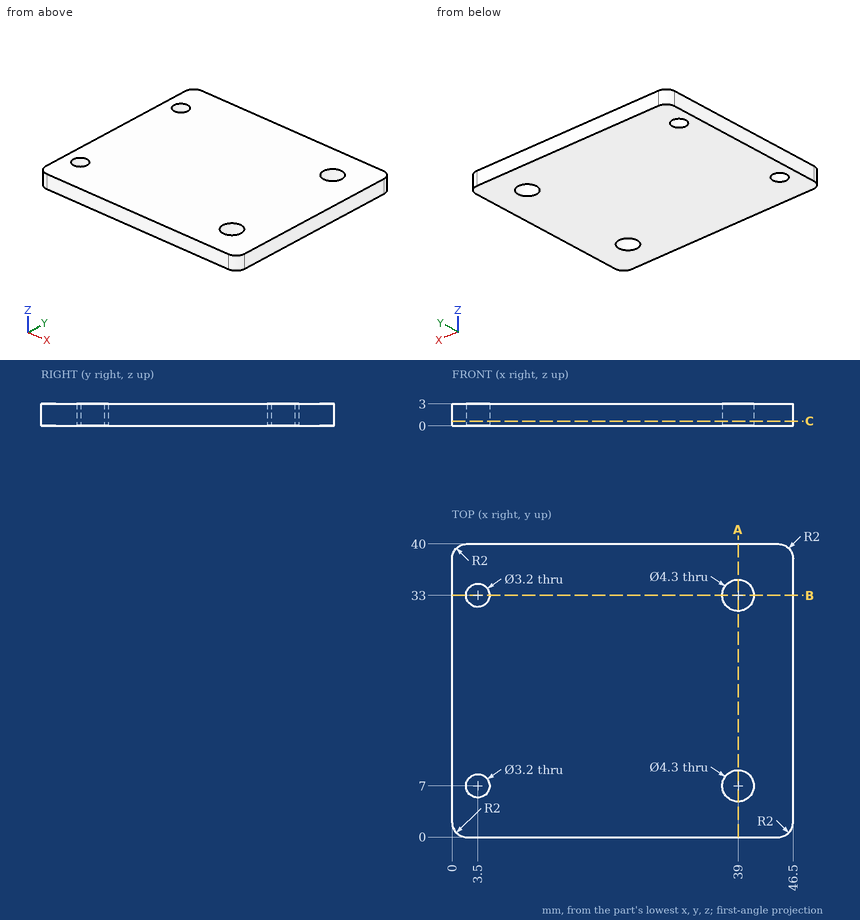
Can you work these out from the drawing? Everything is in mm from the part's minimum corner. Round coordinates to 2 decimals unless told otherwise and drop trailing zeros. Loops run counter-clockwise (first coordinate to the right, second up) from the corner with the lowest first, then second, coordinate; pieces in that order, holes last. Notation, with made-up numbers: (-8, 34.25) -> (0, 34.25) arc R20 ccw to (0, 64.25) -> close; hole circle Ø11 at (-0.75, -9.5). An arc over 180 degrees is marked (long way). One line per question, with ' | ' between items.
(1) If we section it at B-B on y = 33: List the corners of the cut face in (x, z) for me.
Model answer:
outline: (0, 0) -> (1.9, 0) -> (1.9, 3) -> (0, 3) -> close; (5.1, 0) -> (36.85, 0) -> (36.85, 3) -> (5.1, 3) -> close; (41.15, 0) -> (46.5, 0) -> (46.5, 3) -> (41.15, 3) -> close
(2) If I drill on probe 1 along Y at (x, z) = (39, 1.55); probe 2 along Y at (x, z) = (3.5, 0.7); probe 3 along X at (y, z) = (7.5, 0.7), over which ranges is the centre line in solid material (lowest first)?
Model answer:
probe 1: y = 0 to 4.85, 9.15 to 30.85, 35.15 to 40 | probe 2: y = 0 to 5.4, 8.6 to 31.4, 34.6 to 40 | probe 3: x = 0 to 1.98, 5.02 to 36.91, 41.09 to 46.5
(3) If we section it at C-C on z = 0.65: List the corners of the cut face in (x, y) for me.
Model answer:
outline: (0, 2) arc R2 ccw to (2, 0) -> (44.5, 0) arc R2 ccw to (46.5, 2) -> (46.5, 38) arc R2 ccw to (44.5, 40) -> (2, 40) arc R2 ccw to (0, 38) -> close; hole circle Ø3.2 at (3.5, 7); hole circle Ø3.2 at (3.5, 33); hole circle Ø4.3 at (39, 7); hole circle Ø4.3 at (39, 33)
(4) If we section it at A-A on x = 39: List the corners of the cut face in (y, z) for me.
Model answer:
outline: (0, 0) -> (4.85, 0) -> (4.85, 3) -> (0, 3) -> close; (9.15, 0) -> (30.85, 0) -> (30.85, 3) -> (9.15, 3) -> close; (35.15, 0) -> (40, 0) -> (40, 3) -> (35.15, 3) -> close
(5) For pin 1 Ø3.5 at (x, y) = (39, 7) entering from +Z, with a flat end and sliding along its axis, tell me the tip position at first contact or that it passes through.
Model answer:
pin 1: passes through
